from build123d import *

# Parameters (mm, degrees)
F1_R           = 50
F1_R_2         = 45
F1_R_3         = 10
F1_R_4         = 20
F2_DEPTH       = 18
F1_R_5         = 8
F1_R_6         = 4.25
F1_R_7         = 3.5
F3_DEPTH       = 5
F4_DEPTH       = 100
F6_DEPTH       = 50.001
F6_DEPTH_BACK  = 50.001
F9_DEPTH       = 68.3022703266
F9_DEPTH_BACK  = 68.3022703266
F12_DEPTH      = 68.3022703266
F12_DEPTH_BACK = 68.3022703266
F13_SIZE       = 1


with BuildPart() as f2:
    # F1 (on Front) → F2 (new body)
    with BuildSketch(Plane.XZ):
        Circle(F1_R)
        Circle(F1_R_2, mode=Mode.SUBTRACT)
        Circle(F1_R_2)
        with Locations((-29.4448637287, -17)):
            Circle(F1_R_3, mode=Mode.SUBTRACT)
        with Locations((0, -34)):
            Circle(F1_R_3, mode=Mode.SUBTRACT)
        with Locations((29.4448637287, -17)):
            Circle(F1_R_3, mode=Mode.SUBTRACT)
        with Locations((-29.4448637287, 17)):
            Circle(F1_R_3, mode=Mode.SUBTRACT)
        Circle(F1_R_4, mode=Mode.SUBTRACT)
        with Locations((29.4448637287, 17)):
            Circle(F1_R_3, mode=Mode.SUBTRACT)
        with Locations((0, 34)):
            Circle(F1_R_3, mode=Mode.SUBTRACT)
    extrude(amount=-F2_DEPTH)



with BuildPart() as f2b:
    # F1 (on Front) → F2, piece 2 (new body)
    with BuildSketch(Plane.XZ):
        with Locations((-29.4448637287, 17)):
            Circle(F1_R_5)
        with Locations((-29.4448637287, 17)):
            Circle(F1_R_6, mode=Mode.SUBTRACT)
    extrude(amount=-F2_DEPTH)


with BuildPart() as f2c:
    # F1 (on Front) → F2, piece 3 (new body)
    with BuildSketch(Plane.XZ):
        with Locations((0, 34)):
            Circle(F1_R_5)
        with Locations((0, 34)):
            Circle(F1_R_6, mode=Mode.SUBTRACT)
    extrude(amount=-F2_DEPTH)


with BuildPart() as f2d:
    # F1 (on Front) → F2, piece 4 (new body)
    with BuildSketch(Plane.XZ):
        with Locations((29.4448637287, 17)):
            Circle(F1_R_5)
        with Locations((29.4448637287, 17)):
            Circle(F1_R_6, mode=Mode.SUBTRACT)
    extrude(amount=-F2_DEPTH)


with BuildPart() as f2e:
    # F1 (on Front) → F2, piece 5 (new body)
    with BuildSketch(Plane.XZ):
        with Locations((-29.4448637287, -17)):
            Circle(F1_R_5)
        with Locations((-29.4448637287, -17)):
            Circle(F1_R_6, mode=Mode.SUBTRACT)
    extrude(amount=-F2_DEPTH)


with BuildPart() as f2f:
    # F1 (on Front) → F2, piece 6 (new body)
    with BuildSketch(Plane.XZ):
        with Locations((0, -34)):
            Circle(F1_R_5)
        with Locations((0, -34)):
            Circle(F1_R_6, mode=Mode.SUBTRACT)
    extrude(amount=-F2_DEPTH)


with BuildPart() as f2g:
    # F1 (on Front) → F2, piece 7 (new body)
    with BuildSketch(Plane.XZ):
        with Locations((29.4448637287, -17)):
            Circle(F1_R_5)
        with Locations((29.4448637287, -17)):
            Circle(F1_R_6, mode=Mode.SUBTRACT)
    extrude(amount=-F2_DEPTH)


with BuildPart() as f2_1:
    add(f2.part)

    add(f2b.part)  # F3 merges F2b

    add(f2c.part)  # F3 merges F2c

    add(f2d.part)  # F3 merges F2d

    add(f2e.part)  # F3 merges F2e

    add(f2f.part)  # F3 merges F2f

    add(f2g.part)  # F3 merges F2g
    # F1 (on Front) → F3 (join)
    with BuildSketch(Plane.XZ):
        with Locations((0, 34)):
            Circle(F1_R_3)
        with Locations((0, 34)):
            Circle(F1_R_5, mode=Mode.SUBTRACT)
        with Locations((-29.4448637287, 17)):
            Circle(F1_R_3)
        with Locations((-29.4448637287, 17)):
            Circle(F1_R_5, mode=Mode.SUBTRACT)
        with Locations((-29.4448637287, -17)):
            Circle(F1_R_3)
        with Locations((-29.4448637287, -17)):
            Circle(F1_R_5, mode=Mode.SUBTRACT)
        with Locations((0, -34)):
            Circle(F1_R_3)
        with Locations((0, -34)):
            Circle(F1_R_5, mode=Mode.SUBTRACT)
        with Locations((29.4448637287, -17)):
            Circle(F1_R_3)
        with Locations((29.4448637287, -17)):
            Circle(F1_R_5, mode=Mode.SUBTRACT)
        with Locations((29.4448637287, 17)):
            Circle(F1_R_3)
        with Locations((29.4448637287, 17)):
            Circle(F1_R_5, mode=Mode.SUBTRACT)
        with Locations((-29.4448637287, 17)):
            Circle(F1_R_6)
        with Locations((-29.4448637287, 17)):
            Circle(F1_R_7, mode=Mode.SUBTRACT)
        with Locations((0, 34)):
            Circle(F1_R_6)
        with Locations((0, 34)):
            Circle(F1_R_7, mode=Mode.SUBTRACT)
        with Locations((29.4448637287, 17)):
            Circle(F1_R_6)
        with Locations((29.4448637287, 17)):
            Circle(F1_R_7, mode=Mode.SUBTRACT)
        with Locations((-29.4448637287, -17)):
            Circle(F1_R_6)
        with Locations((-29.4448637287, -17)):
            Circle(F1_R_7, mode=Mode.SUBTRACT)
        with Locations((0, -34)):
            Circle(F1_R_6)
        with Locations((0, -34)):
            Circle(F1_R_7, mode=Mode.SUBTRACT)
        with Locations((29.4448637287, -17)):
            Circle(F1_R_6)
        with Locations((29.4448637287, -17)):
            Circle(F1_R_7, mode=Mode.SUBTRACT)
    extrude(amount=-F3_DEPTH)

    # F1 (on Front) → F4 (join)
    with BuildSketch(Plane.XZ):
        Circle(F1_R)
        Circle(F1_R_2, mode=Mode.SUBTRACT)
    extrude(amount=F4_DEPTH)

    # F5 (on Top) → F6 (cut, two sides)
    with BuildSketch(Plane.XY) as f6_sk:
        with BuildLine():
            Line((10, -70), (10, -12))
            ThreePointArc((10, -12), (0, -2), (-10, -12))
            Line((-10, -12), (-10, -70))
            ThreePointArc((-10, -70), (0, -80), (10, -70))
        make_face()
    extrude(amount=-F6_DEPTH, mode=Mode.SUBTRACT)
    extrude(f6_sk.sketch, amount=F6_DEPTH_BACK, mode=Mode.SUBTRACT)

    # F8 (on line) → F9 (cut, two sides)
    with BuildSketch(Plane(origin=(0, 0, 0), x_dir=(0, 1, 0), z_dir=(0.8660254038, 0, -0.5))) as f9_sk:
        with BuildLine():
            Line((-70, -10), (-12, -10))
            ThreePointArc((-12, -10), (-2, 0), (-12, 10))
            Line((-12, 10), (-70, 10))
            ThreePointArc((-70, 10), (-80, 0), (-70, -10))
        make_face()
    extrude(amount=-F9_DEPTH, mode=Mode.SUBTRACT)
    extrude(f9_sk.sketch, amount=F9_DEPTH_BACK, mode=Mode.SUBTRACT)

    # F11 (on line) → F12 (cut, two sides)
    with BuildSketch(Plane(origin=(0, 0, 0), x_dir=(0, -1, 0), z_dir=(-0.8660254038, 0, -0.5))) as f12_sk:
        with BuildLine():
            Line((70, 10), (12, 10))
            ThreePointArc((12, 10), (2, 0), (12, -10))
            Line((12, -10), (70, -10))
            ThreePointArc((70, -10), (80, 0), (70, 10))
        make_face()
    extrude(amount=-F12_DEPTH, mode=Mode.SUBTRACT)
    extrude(f12_sk.sketch, amount=F12_DEPTH_BACK, mode=Mode.SUBTRACT)

    # F13
    f13_edges = [f2_1.edges().sort_by_distance(p)[0] for p in [
        (-45, -100, 0),
        (-50, -100, 0),
        (-50, 18, 0),
    ]]
    chamfer(f13_edges, length=F13_SIZE)


solid = f2_1.part
For this review, take the finished solid that the model builds, in its own axes (mm). A direction names the side the tool comes from. Give positions to 0.01 mm unless a question says otherwise; leave off trailing zeros. Order: outer loops, then holes, each group sorted by start corner. A loop starts at its lowest first (then second) coordinate and runs counter-clockwise, first axis right, second up. Notation, with made-up numbers: (60.25, 40.25) -> (72.25, 40.25) arc R33 ccw to (72.25, 70.25) -> close; hole circle Ø7 at (-12.75, 51.25). An arc over 180 degrees is marked (long way). Write item = value, one per line.
1) We need section C-C, the plane y = -38.5. Give the boundary of the cut face in (x, z), and give its area (3 significant figures).
Findings:
outline = (-47.43, -15.83) -> (-43, -13.28) arc R45 cw to (-43, 13.28) -> (-47.43, 15.83) arc R50 ccw to start; (-37.43, -33.16) arc R50 ccw to (-10, -48.99) -> (-10, -43.87) arc R45 cw to (-33, -30.6) -> close; (-37.43, 33.16) -> (-33, 30.6) arc R45 cw to (-10, 43.87) -> (-10, 48.99) arc R50 ccw to start; (10, -48.99) arc R50 ccw to (37.43, -33.16) -> (33, -30.6) arc R45 cw to (10, -43.87) -> close; (10, 43.87) arc R45 cw to (33, 30.6) -> (37.43, 33.16) arc R50 ccw to (10, 48.99) -> close; (43, -13.28) -> (47.43, -15.83) arc R50 ccw to (47.43, 15.83) -> (43, 13.28) arc R45 cw to start
area = 888 mm^2
2) We need section B-B, the plane z = 0. Give the boundary of the cut face in (x, y).
Findings:
outline = (-50, -99) -> (-49, -100) -> (-46, -100) -> (-45, -99) -> (-45, 0) -> (-20, 0) -> (-20, 18) -> (-49, 18) -> (-50, 17) -> close; (20, 0) -> (45, 0) -> (45, -99) -> (46, -100) -> (49, -100) -> (50, -99) -> (50, 17) -> (49, 18) -> (20, 18) -> close
3) To check wall thickness, follow L1, parallel to Z at x = 0, y = 1; L2, parallel to Y at x = -14, z = -36; L3, parallel to X at y = -58.5, z = 37.5. State the ranges of each line that lie inside material, in increasing order. Write a range as from..to.
Findings:
L1 = -50..-37.5, -30.5..-20, 20..30.5, 37.5..50
L2 = 0..18
L3 = -33.07..-24.87, 24.87..33.07
4) We need section A-A, the plane y = 10.5. Count the separate pieces of the cut face and the enclosed holes in it, and give its area (3 significant figures).
Findings:
separate_pieces = 7
enclosed_holes = 13
area = 5,580 mm^2
5) For faces 1 (the face through (20.765, -59.807, -39.923)), 2 (the face through (-2.17, 11.41, -43.76)), 3 (the face through (40.7, -80, 23.3)), list the 3-axis set-ups (+Z, -Z, +X, -X, +Y, -Y) from which the entire face can be reached by the end or side of a thin tool; tool diameter is ignored.
Findings:
face_1 = -Y
face_2 = +Y
face_3 = none
6) Draft analysis for pull direction Y (two halves, no side actions). For faces 4 (the face through (-40.7, -2, 23.3)), 5 (the face through (-34, 5, 24)), 6 (the face through (-35.79, 11.41, -21.87)), state which applies: pulls with the +Y half, pulls with the -Y half, needs draft (parallel to the pull), parting line crosses it, or undercut.
Findings:
face_4 = undercut
face_5 = pulls with the +Y half
face_6 = needs draft
7) Insertion check: pin 1 (6 mm diameter, centred on y = -8.5, z = 2.5, fed in from -X); pin 2 (12 mm diameter, centred on x = 0, z = -34, fed in from -Y); pin 3 (4 mm diameter, centred on x = -13, y = -28, fed in from -Z) (3 decimals); pin 4 (12 mm diameter, centred on y = -86, z = -21.5, fed in from +X). Each pin has a flat end and moves straight along its axis. Give the tip position at first contact, or say it passes through.
Findings:
pin_1 = -50
pin_2 = 0
pin_3 = -48.775
pin_4 = 47.54
